```python
from build123d import *

# Parameters (mm, degrees)
SKETCH2_R           = 1.55
SKETCH2_R_2         = 1.5
BOSS_EXTRUDE2_DEPTH = 3
SKETCH3_R           = 1.25
SKETCH3_R_2         = 1.5
SKETCH3_R_3         = 1.321701339
CUT_EXTRUDE1_DEPTH  = 10


with BuildPart() as part:
    # Sketch2 → Boss-Extrude2 (new body)
    with BuildSketch(Plane(origin=(0, 0, 0), x_dir=(1, 0, 0), z_dir=(0, 1, 0))):
        with BuildLine():
            Line((-71.018028778, 0), (-80, 0))
            ThreePointArc((-80, 0), (-90, 10), (-80, 20))
            Line((-80, 20), (-71.018028778, 20))
            Line((-71.018028778, 20), (-60, 18))
            ThreePointArc((-60, 18), (-52, 10), (-60, 2))
            Line((-60, 2), (-71.018028778, 0))
        make_face()
        with Locations((-80, 10)):
            Circle(SKETCH2_R, mode=Mode.SUBTRACT)
        with Locations((-60, 10)):
            Circle(SKETCH2_R_2, mode=Mode.SUBTRACT)
    extrude(amount=BOSS_EXTRUDE2_DEPTH)

    # Sketch3 → Cut-Extrude1 (cut)
    with BuildSketch(Plane(origin=(0, 0, 0), x_dir=(1, 0, 0), z_dir=(0, 1, 0))):
        with Locations((-80, 17)):
            Circle(SKETCH3_R)
        with Locations((-80, 3)):
            Circle(SKETCH3_R)
        with Locations((-87, 10)):
            Circle(SKETCH3_R)
        with Locations((-73, 10)):
            Circle(SKETCH3_R)
        with Locations((-66, 10)):
            Circle(SKETCH3_R_2)
        with Locations((-55, 10)):
            Circle(SKETCH3_R_3)
    extrude(amount=CUT_EXTRUDE1_DEPTH, mode=Mode.SUBTRACT)


solid = part.part
```
Geometry: final body of the model. Coordinates: model frame, mm. Round coordinates to 2 decimals unless told otherwise and drop trailing zeros. Order: outer loops, then holes, each group sorted by start corner. A loop starts at its lowest first (then second) coordinate and runs counter-clockwise, first axis right, second up. Notation, with made-up numbers: (-20.75, 33.5) -> (15.25, 33.5) arc R15 cw to (15.25, 54.5) -> close; hole circle Ø7 at (3.5, 84.25). An arc over 180 degrees is marked (long way). Use CSV: the item, a comma, the result in double quotes. Start each with the question number.
1) Material intervals for line 1 along Z through (x, y) = (-80, 1.35); line 2 along Z through (x, y) = (-79, 2.7); line 3 along Z through (x, y) = (-73, 1.85), sorted ascending. Write a range as from..to.
2) First-contact query: pin 1 Ø1.8 at (x, z) = (-60, -10) entering from -Y; pin 2 Ø1.5 at (x, y) = (-67, 2.5) entering from +Z; pin 3 Ø3 at (x, z) = (-80, -17) entering from +Y. Flat tips, straight axial feed; report the tip coordinate or a pass-through.
3) Section B-B (y = 1.9). State how many separate pieces and enclosed holes the cut face has, and give its area (3 significant figures).
4) Section A-A (x = -73). Return the cut outline in (y, z), and give its area (3 significant figures).
5) Section C-C (x = -66). Return the cut outline in (y, z).
6) Draft query along X for faces 1 (the face through (-90, 1, -10)), 2 (the face through (-71.81, 1.48, -10.38)), 3 (the face through (-76, 1, -20)), 4 (the face through (-52, 1, -10)). Return one class per face: +X half, -X half, draft (parallel to the pull), parting line (faces both ways), or undercut.
7) Section D-D (z = -6). Return the cut outline in (x, y), and give its area (3 significant figures).
Returned:
1,line 1,"z = -20..-18.25, -15.75..-11.55, -8.45..-4.25, -1.75..0"
1,line 2,"z = -20..-17.75, -16.25..-11.18, -8.82..-3.75, -2.25..0"
1,line 3,"z = -20..-11.25, -8.75..0"
2,pin 1,"passes through"
2,pin 2,"stops at z = -0.59"
2,pin 3,"stops at y = 3"
3,separate pieces,"1"
3,enclosed holes,"8"
3,area,"589 mm²"
4,outline,"(0, -20) -> (3, -20) -> (3, -11.25) -> (0, -11.25) -> close; (0, -8.75) -> (3, -8.75) -> (3, 0) -> (0, 0) -> close"
4,area,"52.5 mm²"
5,outline,"(0, -19.09) -> (3, -19.09) -> (3, -11.5) -> (0, -11.5) -> close; (0, -8.5) -> (3, -8.5) -> (3, -0.91) -> (0, -0.91) -> close"
6,face 1,"-X half"
6,face 2,"undercut"
6,face 3,"draft"
6,face 4,"+X half"
7,outline,"(-89.17, 0) -> (-53.07, 0) -> (-53.07, 3) -> (-89.17, 3) -> close"
7,area,"108 mm²"
